```python
from build123d import *

# Parameters (mm, degrees)
F1_DEPTH = 254
F2_DEPTH = 228.6


with BuildPart() as f1:
    # F0 (on Front) → F1 (new body)
    with BuildSketch(Plane.XZ):
        with BuildLine():
            ThreePointArc((-39.860837, 56.103354), (-44.462967, 33.7664), (-23.985837, 43.806632))
            ThreePointArc((-23.985837, 43.806632), (-26.645606, 51.583762), (-33.510837, 56.103354))
            ThreePointArc((-33.510837, 56.103354), (-35.085583, 56.405409), (-36.685837, 56.506632))
            ThreePointArc((-36.685837, 56.506632), (-38.286092, 56.405409), (-39.860837, 56.103354))
        make_face()
    extrude(amount=F1_DEPTH)

    # F0 (on Front) → F2 (join)
    with BuildSketch(Plane.XZ):
        with BuildLine():
            Line((-39.860837, 59.681632), (-39.860837, 56.103354))
            ThreePointArc((-39.860837, 56.103354), (-38.286092, 56.405409), (-36.685837, 56.506632))
            Line((-36.685837, 56.506632), (-36.685837, 59.681632))
            Line((-36.685837, 59.681632), (-39.860837, 59.681632))
        make_face()
        with BuildLine():
            ThreePointArc((-36.685837, 56.506632), (-35.085583, 56.405409), (-33.510837, 56.103354))
            Line((-33.510837, 56.103354), (-33.510837, 59.681632))
            Line((-33.510837, 59.681632), (-36.685837, 59.681632))
            Line((-36.685837, 59.681632), (-36.685837, 56.506632))
        make_face()
    extrude(amount=F2_DEPTH)


solid = f1.part
```
Geometry: final body of the model. Coordinates: model frame, mm. Give positions to 0.01 mm unless a question says otherwise; leave off trailing zeros. Write each loop counter-clockwise with the first axis right and the second up, starting at its lowest first coordinate (ties: lowest second). Pieces come first, ordered by that corner, then holes.
1. Section query B-B, the plane z = 50.5. Return loops of the section in (x, y), then the cut area to 3 significant figures.
2. Pin query (flat end, axial travel): P1, Ø4, axis at x = -26.5, y = -228.5, coming from the +Z side; P2, Ø4, axis at y = -153, z = 58.5, coming from the +X side; P3, Ø10, axis at x = -45.5, y = -84.5, coming from the -Z side. Return the tip coordinate at first contact, or that it passes through.
3. Section query C-C, the plane x = -31.25. Return loops of the section in (y, z).
4. Section query A-A, the plane y = -99.5. Return loops of the section in (x, z), then the cut area to 3 significant figures.
5. Line query: probe 1 along X at (y, z) = (-78, 57); probe 2 along X at (y, z) = (-124, 42.75); probe 3 along Z at (x, y) = (-36.25, -167.5). Output: solid intervals per line, ascending.
Computed:
1. outline: (-47.48, -254) - (-25.89, -254) - (-25.89, 0) - (-47.48, 0) - close
1. area: 5,480 mm2
2. P1: stops at z = 53.52
2. P2: stops at x = -33.51
2. P3: stops at z = 31.69
3. outline: (-254, 32.33) - (0, 32.33) - (0, 55.28) - (-254, 55.28) - close
4. outline: (-39.86, 56.1) arc R12.7 ccw (long way) to (-23.99, 43.81) arc R12.7 ccw to (-33.51, 56.1) - (-33.51, 59.68) - (-39.86, 59.68) - close
4. area: 528 mm2
5. probe 1: x = -39.86 to -33.51
5. probe 2: x = -49.34 to -24.03
5. probe 3: z = 31.11 to 59.68
